The figure shows three views and two pictorial views of one solid part (mm, origin at its lowest corner). Answer the questions. A direction names the side the tool comes from. Coordinates: 2 decimals unless noted, no trailing zeros. Order: outer loops, then holes, each group sorted by start corner. A loop starts at its lowest first (then second) coordinate and runs counter-clockwise, first axis right, second up. Notation, with made-up numbers: (-23, -6.75) -> (19, -6.75) arc R30 ccw to (19, 17.25) -> close; hole circle Ø7 at (38, 28.25). An arc over 180 degrees is marked (long way). Write item = value, one per line. Start each with the question number.
Q1. The part is cut by section A-A, the plane y = 5. Determine the outline of the cut face in (x, z) (3 decimals).
Q2. The part is cut by section C-C, the plane z = 20.5. Determine the outline of the cut face in (x, y) (3 decimals), plus the area to 3 significant figures.
Q3. Straight lines are drawn through the part: L1, parallel to Y at x = 5, z = 33.5 (3 decimals); L2, parallel to Z at x = 1.5, y = 2; L3, parallel to X at y = 6.25, z = 34.5. For each, find the intervals that lie inside material, in ascending order. Write a range as from..to.
Q4. Which of the six approach directions +Z, -Z, +X, -X, +Y, -Y give full straight-line access (tool end or side, diameter ignored) to the marked faces 1 and 2?
Q5. Flat-ended cylindrical pins translate along their axes: pin 1 (6 mm diameter, centred on x = 6, z = 17, fed in from +Y) (3 decimals); pin 2 (2 mm diameter, centred on y = 2, z = 21.5, fed in from -X); pin 3 (1 mm diameter, centred on y = 1.5, z = 34, fed in from +X); pin 4 (0.9 mm diameter, centred on x = 5.5, y = 4.5, fed in from +Z). Find the tip coordinate at first contact, or state that the pin passes through.
Q6. The part is cut by section D-D, the plane y = 2. Determine the outline of the cut face in (x, z).
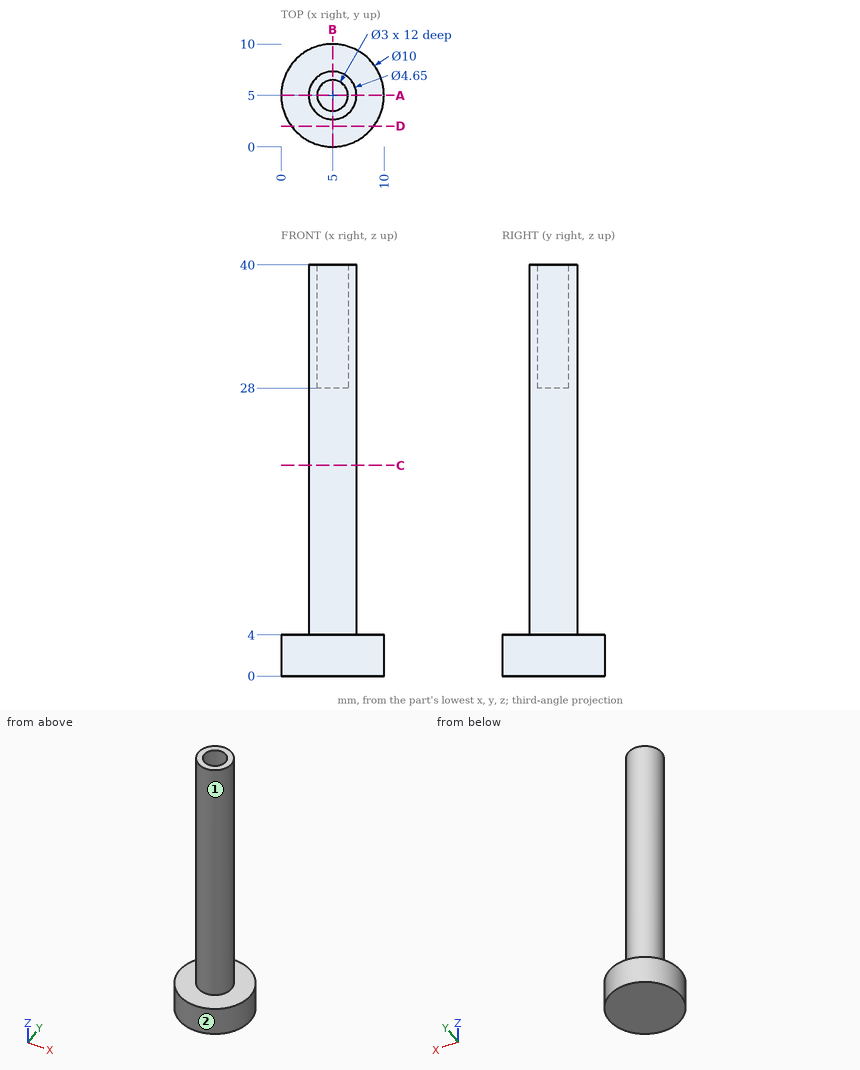
Model answer:
q1.outline = (0, 0) -> (10, 0) -> (10, 4) -> (7.325, 4) -> (7.325, 40) -> (6.5, 40) -> (6.5, 28) -> (3.5, 28) -> (3.5, 40) -> (2.675, 40) -> (2.675, 4) -> (0, 4) -> close
q2.outline = circle Ø4.65 at (5, 5)
q2.area = 17.0 mm2
q3.L1 = 2.675..3.5, 6.5..7.325
q3.L2 = 0..4
q3.L3 = 3.04..4.17, 5.83..6.96
q4.face_1 = +Z
q4.face_2 = +Z, -Z
q5.pin_1 = 7.325
q5.pin_2 = 3.81
q5.pin_3 = through
q5.pin_4 = 28
q6.outline = (1, 0) -> (9, 0) -> (9, 4) -> (1, 4) -> close
